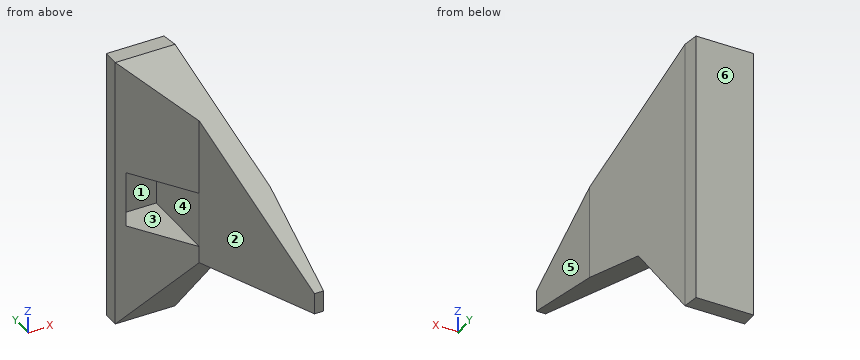
```python
from build123d import *

# Parameters (mm, degrees)
SKETCH_1_W               = 20
SKETCH_1_H               = 70
EXTRUDE_1_DEPTH          = 68
SKETCH_2_W               = 10.341057985
SKETCH_2_H               = 14.244474777
CUT_EXTRUDE_1_DEPTH      = 66.5
CUT_EXTRUDE_2_DEPTH      = 27
CUT_EXTRUDE_2_DEPTH_BACK = 28.5
CUT_EXTRUDE_3_DEPTH      = 18
CUT_EXTRUDE_3_DEPTH_BACK = 80.5


with BuildPart() as part:
    # 草图1 → 凸台-拉伸1 (new body)
    with BuildSketch(Plane(origin=(0, 0, 0), x_dir=(1, 0, 0), z_dir=(0, 1, 0))):
        Rectangle(SKETCH_1_W, SKETCH_1_H)
    extrude(amount=EXTRUDE_1_DEPTH)

    # 草图2 → 切除-拉伸1 (cut)
    with BuildSketch(Plane.XZ):
        with Locations((-3.329471008, -0.802163256)):
            Rectangle(SKETCH_2_W, SKETCH_2_H)
    extrude(amount=-CUT_EXTRUDE_1_DEPTH, mode=Mode.SUBTRACT)

    # 草图3 → 切除-拉伸2 (cut, two sides)
    with BuildSketch(Plane.ZY.offset(10)) as cut_extrude_2_sk:
        Polygon((-35, 68), (-35, 63.923584322), (-12.228951857, 46.66952319), (-2.701261913, 4.015150281), (2.701261913, 4.015150281), (35, 63.923584322), (35, 68), (43.781903243, 68), (43.781903243, -5.043476458), (-39.089851198, -5.043476458), (-39.089851198, 68), align=None)
    extrude(amount=CUT_EXTRUDE_2_DEPTH, mode=Mode.SUBTRACT)
    extrude(cut_extrude_2_sk.sketch, amount=-CUT_EXTRUDE_2_DEPTH_BACK, mode=Mode.SUBTRACT)

    # 草图4 → 切除-拉伸3 (cut, two sides)
    with BuildSketch(Plane(origin=(0, 0, -35), x_dir=(-1, 0, 0), z_dir=(0, 0, -1))) as cut_extrude_3_sk:
        Polygon((-10, 28.610295414), (-5.14861474, 63.923584322), (-10, 63.923584322), align=None)
        Polygon((-5.14861474, 63.923584322), (-4.588591487, 68), (-10, 68), (-10, 63.923584322), align=None)
        Polygon((-7.700970851, -1.077719905), (-7.700970851, 4.015150281), (-1.841057985, 46.66952319), (10, 63.923584322), (16.463180064, 63.923584322), (16.463180064, -1.077719905), align=None)
    extrude(amount=CUT_EXTRUDE_3_DEPTH, mode=Mode.SUBTRACT)
    extrude(cut_extrude_3_sk.sketch, amount=-CUT_EXTRUDE_3_DEPTH_BACK, mode=Mode.SUBTRACT)


solid = part.part
```
Design review of the part built by this model. Coordinates are the model's own, in mm. Face numbers are marked on the shaded views. A direction names the side the tool comes from. Give positions to 0.01 mm unless a question says otherwise; leave off trailing zeros. Write each loop counter-clockwise with the first axis right and the second up, starting at its lowest first coordinate (ties: lowest second). Pieces come first, ordered by that corner, then holes.
(1) Mouldability with a two-part tool opening along X and no side actions: class the marked faces 3, 4, 5 and 6 as +X half, -X half, draft (parallel to the pull), parting line (faces both ways), or undercut.
Checked values:
face 3: undercut
face 4: undercut
face 5: +X half
face 6: draft
(2) Add section D-D (z = -6.5). Give the boundary of the cut face in (x, y), and give its area (3 significant figures).
Checked values:
outline: (-10, 63.92) - (-8.5, 61.74) - (-8.5, 66.5) - (1.84, 66.5) - (1.84, 46.67) - (5.36, 21.02) - (10, 21.02) - (10, 28.61) - (4.59, 68) - (-10, 68) - close
area: 255 mm2
(3) Wall thickness on line 1 along Y through (x, z) = (-6.75, 4.5); line 2 along X through (y, z) = (65, 3); line 3 along Z through (x, y) = (-2.5, 56.5): over which ranges is each line inside the solid? List them lowest first.
Checked values:
line 1: y = 66.5 to 68
line 2: x = -10 to -8.5, 1.84 to 5
line 3: z = -25.2 to -7.92, 6.32 to 31
(4) Tool access review of the marked faces 1 and 2: name each direction out of +Z, -Z, +X, -X, +Y, -Y from which nothing blocks a thin tool from reaching the whole face with its end or side.
Checked values:
face 1: -Y
face 2: +Z, -Z, -X, -Y
(5) Add section C-C (z = 13.5). Give the boundary of the cut face in (x, y), and give its area (3 significant figures).
Checked values:
outline: (-10, 63.92) - (1.84, 46.67) - (4.95, 24.04) - (10, 24.04) - (10, 28.61) - (4.59, 68) - (-10, 68) - close
area: 367 mm2
(6) Clearance check with flat-ended pins moving along their axes: pin 1 Ø3 at (x, z) = (-5.5, -2.5) entering from -Y; pin 2 Ø10 at (x, y) = (5, 50.5) entering from -Z; pin 3 Ø5 at (y, z) = (44.5, 15) entering from +X; pin 4 Ø4 at (x, y) = (2, 30) entering from -Z. State where each tip first meets the part, or that it passes through.
Checked values:
pin 1: stops at y = 66.5
pin 2: stops at z = -23.88
pin 3: stops at x = 8.16
pin 4: passes through
(7) Add section B-B (y = 55.5). Give the boundary of the cut face in (x, z), and give its area (3 significant figures).
Checked values:
outline: (-4.22, -23.88) - (6.31, -23.88) - (6.31, 30.46) - (-4.22, 30.46) - (-4.22, 6.32) - (1.84, 6.32) - (1.84, -7.92) - (-4.22, -7.92) - close
area: 486 mm2
(8) Add section A-A (x = -0.25). Give the boundary of the cut face in (y, z).
Checked values:
outline: (49.72, -16.25) - (63.92, -35) - (68, -35) - (68, 35) - (63.92, 35) - (49.72, 27.34) - (49.72, 6.32) - (66.5, 6.32) - (66.5, -7.92) - (49.72, -7.92) - close
